```python
from build123d import *

# Parameters (mm, degrees)
SKETCH1_W                                       = 82.6
SKETCH1_H                                       = 98
SKETCH1_R                                       = 1.6
SKETCH1_W_2                                     = 19.8
SKETCH1_H_2                                     = 3.7
SKETCH1_W_3                                     = 17.672668113
SKETCH1_W_4                                     = 15.589154013
BOSS_EXTRUDE1_DEPTH                             = 1.6
SKETCH1_3_W                                     = 17.672668113
SKETCH1_3_H                                     = 3.7
SKETCH1_3_W_2                                   = 15.589154013
SKETCH1_3_W_3                                   = 19.8
BOSS_EXTRUDE2_DEPTH                             = 1.6
SKETCH2_W                                       = 68.729308582
SKETCH2_H                                       = 32.090135436
SKETCH2_H_2                                     = 34.029409061
BOSS_EXTRUDE3_DEPTH                             = 0.4
CSK_FOR_M3_FLAT_HEAD_MACHINE_SCREW1_D           = 3.4
CSK_FOR_M3_FLAT_HEAD_MACHINE_SCREW1_DEPTH       = 3.15
CSK_FOR_M3_FLAT_HEAD_MACHINE_SCREW1_CSINK_D     = 6.3
CSK_FOR_M3_FLAT_HEAD_MACHINE_SCREW1_CSINK_ANGLE = 90
CSK_FOR_M3_FLAT_HEAD_MACHINE_SCREW1_TIP         = 1.021463052


with BuildPart() as part:
    # Sketch1 → Boss-Extrude1 (new body)
    # profile 1 of 4: a face of its own
    with BuildSketch(Plane(origin=(0, 0, 0), x_dir=(1, 0, 0), z_dir=(0, 1, 0))):
        Rectangle(SKETCH1_W, SKETCH1_H)
        with Locations(Location((38.1, -45.8, 0), (0, 0, 270))):
            Circle(SKETCH1_R, mode=Mode.SUBTRACT)
        with Locations(Location((38.1, 45.8, 0), (0, 0, 270))):
            Circle(SKETCH1_R, mode=Mode.SUBTRACT)
        with Locations(Location((-38.1, -45.8, 0), (0, 0, 270))):
            Circle(SKETCH1_R, mode=Mode.SUBTRACT)
        with Locations(Location((-38.1, 45.8, 0), (0, 0, 270))):
            Circle(SKETCH1_R, mode=Mode.SUBTRACT)
        with Locations((-4.972668113, -38.05)):
            Rectangle(SKETCH1_W_2, SKETCH1_H_2, mode=Mode.SUBTRACT)
        with Locations((15.263665944, -38.05)):
            Rectangle(SKETCH1_W_3, SKETCH1_H_2, mode=Mode.SUBTRACT)
        with Locations((16.305422994, -32.85)):
            Rectangle(SKETCH1_W_4, SKETCH1_H_2, mode=Mode.SUBTRACT)
    # profile 2 of 4: a face of its own
    with BuildSketch(Plane(origin=(0, 0, 0), x_dir=(1, 0, 0), z_dir=(0, 1, 0))):
        with Locations((15.263665944, -38.05)):
            Rectangle(SKETCH1_W_3, SKETCH1_H_2)
    # profile 3 of 4: a face of its own
    with BuildSketch(Plane(origin=(0, 0, 0), x_dir=(1, 0, 0), z_dir=(0, 1, 0))):
        with Locations((16.305422994, -32.85)):
            Rectangle(SKETCH1_W_4, SKETCH1_H_2)
    # profile 4 of 4: a face of its own
    with BuildSketch(Plane(origin=(0, 0, 0), x_dir=(1, 0, 0), z_dir=(0, 1, 0))):
        with Locations((-4.972668113, -38.05)):
            Rectangle(SKETCH1_W_2, SKETCH1_H_2)
    extrude(amount=BOSS_EXTRUDE1_DEPTH)

    # Sketch1_3 → Boss-Extrude2 (add)
    with BuildSketch(Plane(origin=(0, 0, 0), x_dir=(1, 0, 0), z_dir=(0, 1, 0))):
        with Locations((15.263665944, -38.05)):
            Rectangle(SKETCH1_3_W, SKETCH1_3_H)
        with Locations((16.305422994, -32.85)):
            Rectangle(SKETCH1_3_W_2, SKETCH1_3_H)
        with Locations((-4.972668113, -38.05)):
            Rectangle(SKETCH1_3_W_3, SKETCH1_3_H)
    extrude(amount=-BOSS_EXTRUDE2_DEPTH)

    # Sketch2 → Boss-Extrude3 (add)
    with BuildSketch(Plane(origin=(0, 1.6, 0), x_dir=(1, 0, 0), z_dir=(0, 1, 0))):
        with Locations((0, 31.074476779)):
            Rectangle(SKETCH2_W, SKETCH2_H)
        with Locations((0, -16.985295469)):
            Rectangle(SKETCH2_W, SKETCH2_H_2)
    extrude(amount=BOSS_EXTRUDE3_DEPTH)

    # CSK for M3 Flat Head Machine Screw1
    with Locations(Plane(origin=(0, 1.6, 0), x_dir=(1, 0, 0), z_dir=(0, 1, 0))):
        with Locations((-38.1, 45.8), (38.1, 45.8), (38.1, -45.8), (-38.1, -45.8)):
            CounterSinkHole(CSK_FOR_M3_FLAT_HEAD_MACHINE_SCREW1_D / 2, CSK_FOR_M3_FLAT_HEAD_MACHINE_SCREW1_CSINK_D / 2, depth=CSK_FOR_M3_FLAT_HEAD_MACHINE_SCREW1_DEPTH, counter_sink_angle=CSK_FOR_M3_FLAT_HEAD_MACHINE_SCREW1_CSINK_ANGLE)
            with Locations((0, 0, -(CSK_FOR_M3_FLAT_HEAD_MACHINE_SCREW1_DEPTH + CSK_FOR_M3_FLAT_HEAD_MACHINE_SCREW1_TIP / 2))):  # 118° drill point
                Cone(0, CSK_FOR_M3_FLAT_HEAD_MACHINE_SCREW1_D / 2, CSK_FOR_M3_FLAT_HEAD_MACHINE_SCREW1_TIP, mode=Mode.SUBTRACT)


solid = part.part
```
The listing builds one solid part. Answer for the finished solid, in the listing's coordinates (mm). Round coordinates to 2 decimals unless told otherwise and drop trailing zeros. Order: outer loops, then holes, each group sorted by start corner. A loop starts at its lowest first (then second) coordinate and runs counter-clockwise, first axis right, second up. Notation, with made-up numbers: (45, 78.25) - (90, 78.25) arc R19 cw to (90, 99.25) - close; hole circle Ø6 at (31.5, 68.25). An arc over 180 degrees is marked (long way). Put each result on its own line as item: value. Start each with the question number.
(1) Find section D-D (x = 1). Give the vertices of the cut face in (y, z), plus the area to 3 significant figures.
(2) Find section A-A (x = -38.1). Give the vertices of the cut face in (y, z), plus the area to 3 significant figures.
(3) Straight lines are drawn through the part: probe 1 along Z at (x, y) = (38.1, 0.1); probe 2 along X at (y, z) = (0.05, -45.8); probe 3 along Z at (x, y) = (-1.5, 1.8). For each, find the intervals that lie inside material, in ascending order. Write a range as from..to.
(4) Find section B-B (y = -0.75). Give the vertices of the cut face in (x, z), plus the area to 3 significant figures.
(5) Given P1, Ø0.5, axis at y = -1, z = 39, coming from the -X side; P2, Ø1.3, axis at x = 16, y = -1, coming from the +Z side; P3, Ø1.3, axis at y = -0.5, z = 39, coming from the -X side; P4, Ø10, axis at x = 27, z = 25, coming from the -Y side, each flat-ended and moving along its own axis, determine where each tip first touches the part or whether it passes through.
(6) Find section C-C (z = -45.8). Give the vertices of the cut face in (x, y), plus the area to 3 significant figures.
Reply:
1. outline: (-1.6, 36.2) - (0, 36.2) - (0, -49) - (1.6, -49) - (1.6, -47.12) - (2, -47.12) - (2, -15.03) - (1.6, -15.03) - (1.6, -0.03) - (2, -0.03) - (2, 34) - (1.6, 34) - (1.6, 49) - (0, 49) - (0, 39.9) - (-1.6, 39.9) - close
1. area: 189 mm^2
2. outline: (0, -49) - (1.6, -49) - (1.6, -48.95) - (0.15, -47.5) - (0, -47.5) - close; (0, -44.1) - (0.15, -44.1) - (1.6, -42.65) - (1.6, 42.65) - (0.15, 44.1) - (0, 44.1) - close; (0, 47.5) - (0.15, 47.5) - (1.6, 48.95) - (1.6, 49) - (0, 49) - close
2. area: 142 mm^2
3. probe 1: -49..-47.5, -44.1..44.1, 47.5..49
3. probe 2: -41.3..-39.8, -36.4..36.4, 39.8..41.3
3. probe 3: -47.12..-15.03, -0.03..34
4. outline: (-14.87, 36.2) - (4.93, 36.2) - (4.93, 39.9) - (-14.87, 39.9) - close; (6.43, 36.2) - (24.1, 36.2) - (24.1, 39.9) - (6.43, 39.9) - close; (8.51, 31) - (24.1, 31) - (24.1, 34.7) - (8.51, 34.7) - close
4. area: 196 mm^2
5. P1: x = -14.87
5. P2: z = 39.9
5. P3: x = -41.3
5. P4: y = 0
6. outline: (-41.3, 0) - (-39.8, 0) - (-39.8, 0.15) - (-41.25, 1.6) - (-41.3, 1.6) - close; (-36.4, 0) - (36.4, 0) - (36.4, 0.15) - (34.95, 1.6) - (34.36, 1.6) - (34.36, 2) - (-34.36, 2) - (-34.36, 1.6) - (-34.95, 1.6) - (-36.4, 0.15) - close; (39.8, 0) - (41.3, 0) - (41.3, 1.6) - (41.25, 1.6) - (39.8, 0.15) - close
6. area: 145 mm^2
